Design review of the part built by this model. Coordinates are the model's own, in mm. A direction names the side the tool comes from. Coordinates: 2 decimals unless noted, no trailing zeros. Order: outer loops, then holes, each group sorted by start corner. A loop starts at its lowest first (then second) coordinate and runs counter-clockwise, first axis right, second up. Notation, with made-up numbers: (21, 74) -> (35, 74) arc R20 ccw to (35, 108) -> close; hole circle Ø7 at (62, 21.5). An arc over 180 degrees is marked (long way). Write item = value, one per line.
Autodesk Inventor part; units mm, degrees
ref_plane "YZ Plane" through (0, 0, 0) normal (1, 0, 0) x (0, 1, 0)
ref_plane "XZ Plane" through (0, 0, 0) normal (0, 1, 0) x (-1, 0, 0)
ref_plane "XY Plane" through (0, 0, 0) normal (0, 0, 1) x (1, 0, 0)
sketch "Sketch1" plane through (0, 0, 0) normal (0, 0, 1) x (1, 0, 0)
  circle A0 centre (0, 0) radius 17.75
  dimension "d0" = 35.5
extrude "Extrusion1" add sketch "Sketch1" along normal blind 16.8
sketch "Sketch2" plane through (0, 0, 16.8) normal (0, 0, 1) x (1, 0, 0)
  circle A0 centre (0, 0) radius 17.75
  circle A1 centre (0, 0) radius 18.25
  dimension "d3" = 36.5
extrude "Extrusion2" add sketch "Sketch2" along normal blind 14.7 contours A0 | A1
chamfer "Chamfer1" distance 3 distance2 12 1 edges at (-17.75, 0, 0) measured on face at (-0.7132, -5.1908, 0)
sketch "Sketch3" plane through (0, 0, 31.5) normal (0, 0, 1) x (1, 0, 0)
  circle A0 centre (0, 0) radius 18.25
  circle A1 centre (0, 0) radius 17.75
  dimension "d9" = 35.5
extrude "Extrusion3" add sketch "Sketch3" along normal blind 2.8 contours A1
sketch "Sketch4" plane through (0, 0, 34.3) normal (0, 0, 1) x (1, 0, 0)
  circle A0 centre (0, 0) radius 17.75
  circle A1 centre (0, 0) radius 18.25
  dimension "d12" = 36.5
extrude "Extrusion4" add sketch "Sketch4" along normal blind 25.25 contours A0 | A1
sketch "Sketch5" plane through (0, 0, 59.55) normal (0, 0, 1) x (1, 0, 0)
  circle A0 centre (0, 0) radius 18.25
  circle A1 centre (0, 0) radius 17.75
  dimension "d15" = 35.5
extrude "Extrusion5" add sketch "Sketch5" along normal blind 1 contours A1
sketch "Sketch6" plane through (0, 0, 60.55) normal (0, 0, 1) x (1, 0, 0)
  circle A0 centre (0, 0) radius 17.75
  circle A1 centre (0, 0) radius 18.25
  dimension "d18" = 36.5
extrude "Extrusion6" add sketch "Sketch6" along normal blind 13.2 contours A0 | A1
sketch "Sketch7" plane through (0, 0, 73.75) normal (0, 0, 1) x (1, 0, 0)
  circle A0 centre (0, 0) radius 18.25
  circle A1 centre (0, 0) radius 17.75
  dimension "d21" = 35.5
extrude "Extrusion7" add sketch "Sketch7" along normal blind 1 contours A1
sketch "Sketch8" plane through (0, 0, 74.75) normal (0, 0, 1) x (1, 0, 0)
  circle A0 centre (0, 0) radius 17.75
  circle A1 centre (0, 0) radius 18.25
  dimension "d24" = 36.5
extrude "Extrusion8" add sketch "Sketch8" along normal blind 4.85 contours A0 | A1
sketch "Sketch9" plane through (0, 0, 79.6) normal (0, 0, 1) x (1, 0, 0)
  circle A0 centre (0, 0) radius 16.9026
extrude "Extrusion9" cut sketch "Sketch9" against normal blind 3
properties part number "MLM3X-MP" material "Acetal Resin, Black"
(1) For faces 4 (the flat face through (4, -17.5, 34.3)), 5 (the cylindrical face through (-13.4, -10.3, 78.1)), 6 (the flat face through (0, 0, 0)), 7 (the cylindrical face through (-3.956, 17.816, 77.141)), 8 (the flat face through (4, -17.5, 16.8)), list the 3-axis set-ups (+Z, -Z, +X, -X, +Y, -Y) from which the entire face can be reached by the end or side of a thin tool; tool diameter is ignored.
Report:
face_4 = none
face_5 = +Z
face_6 = -Z, +X, -X, +Y, -Y
face_7 = +Z, -Z
face_8 = -Z
(2) Insertion check: pin 1 (4 mm diameter, centred on y = 10.5, z = 41.5, fed in from +X); pin 2 (1 mm diameter, centred on x = 1, y = -10.5, fed in from +Z); pin 3 (18 mm diameter, centred on x = 6.5, y = -1.5, fed in from -Z); pin 4 (8 mm diameter, centred on x = -6, z = 57, fed in from -Y). Each pin has a flat end and moves straight along its axis. Give the tip position at first contact, or say it passes through.
Report:
pin_1 = 16.15
pin_2 = 76.6
pin_3 = 0
pin_4 = -18.14
(3) We need section A-A (z = 21.5). Write out the cut boundary in (x, y).
Report:
outline = circle Ø36.5 at (0, 0)
(4) The part is to be moulded in two halves that separate along Z. For faces 1 (the cylindrical face through (-3.848, 17.328, 32.88)), 2 (the conical face through (-3.31, -14.908, 2.084)), 3 (the cylindrical face through (-3.848, 17.328, 14.366)), say which applies: released by +Z, released by -Z, zero draft, split by the parting line, or undercut.
Report:
face_1 = undercut
face_2 = released by -Z
face_3 = zero draft
(5) For L1, parallel to Y at x = 0, z = 77.75; L2, parallel to Z at x = -8, y = 16; L3, parallel to Z at x = 13, y = -5.5, list the stretches that pass through material, from the lowest coordinate up.
Report:
L1 = -18.25 to -16.9, 16.9 to 18.25
L2 = 16.8 to 31.5, 34.3 to 59.55, 60.55 to 73.75, 74.75 to 79.6
L3 = 0 to 76.6
